Can you work these out from the drawing? Everything is in mm from the part's minimum corner. A direction names the side the tool comes from. Round coordinates to 2 decimals unless told otherwise and drop trailing zeros. Write each loop counter-clockwise with the first axis right and the second up, starting at its lowest first coordinate (ties: lowest second). Pieces come first, ordered by that corner, then holes. Notation, with made-up numbers: M 23.25,-13.5 L 36.25,-13.5 A24 cw 36.25,7.5 Z; hole C 16.5,-17.75 d9. An arc over 180 degrees is marked long. Use one line per item in the form item = value. Start each with the question number.
Q1. I want a section at A-A on y = 24. List the corners of the cut face in (x, z) for me.
Q2. I'm going to push flat-ended pins straight in: pin 1 Ø10 at (y, z) = (11, 7.5) entering from +X; pin 2 Ø2 at (y, z) = (27.5, 7) entering from +X; pin 3 Ø3 at (x, z) = (23.5, 8.5) entering from +Y (1 decimal). Where does each tip first touch, or does it pass through?
Q3. I want a section at C-C on z = 9.25. List the corners of the cut face in (x, y) for me, and give its area (3 significant figures).
Q4. I want a section at B-B on x = 23. List the corners of the cut face in (y, z) for me (1 decimal).
Q5. We'd pull the mould along X, two halves only. Please class the marked faces 3, 4 and 5: +X half, -X half, draft (parallel to the pull), parting line (faces both ways), or undercut.
Q6. For the marked faces 1 and 2, which set-ups out of +Z, -Z, +X, -X, +Y, -Y let a thin tool reach every point of the face, with its end or its side?
Q7. I need wall thicknesses on line 1 along X through (y, z) = (29.5, 8.5) (1 decimal); line 2 along X through (y, z) = (17, 10.25) (1 decimal); line 3 along Y through (x, z) = (19, 14.25). Which ranges of each line are inside material? Lowest first, please. Write a range as from..to.
Q8. I want a section at D-D on y = 13. List the corners of the cut face in (x, z) for me, and give its area (3 significant figures).
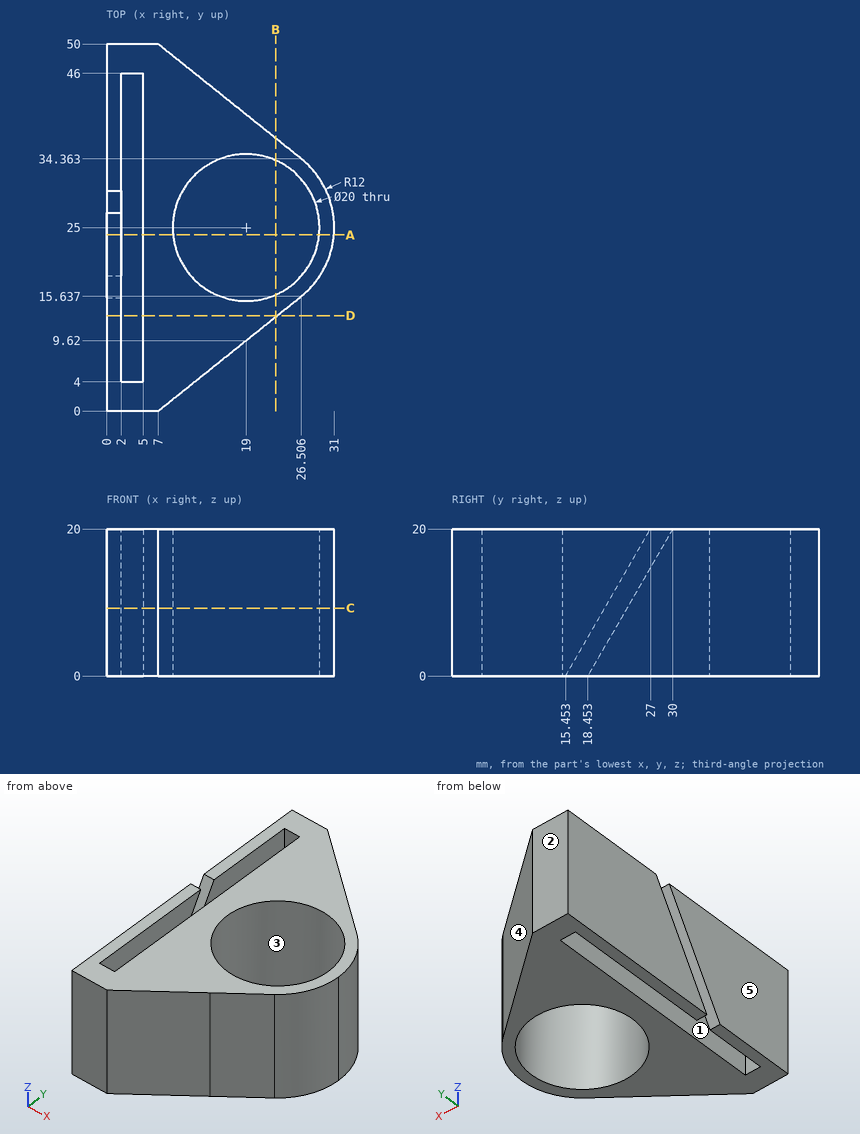
Reported:
q1.outline = M 0,0 L 2,0 L 2,9.61 L 0,9.61 Z; M 0,14.8 L 2,14.8 L 2,20 L 0,20 Z; M 5,0 L 9.05,0 L 9.05,20 L 5,20 Z; M 28.95,0 L 30.96,0 L 30.96,20 L 28.95,20 Z
q2.pin_1 = 26.94
q2.pin_2 = 30.91
q2.pin_3 = 38
q3.outline = M 0,0 L 7,0 L 26.51,15.64 A12 ccw 26.51,34.36 L 7,50 L 0,50 L 0,23.79 L 2,23.79 L 2,46 L 5,46 L 5,4 L 2,4 L 2,20.79 L 0,20.79 Z; hole C 19,25 d20
q3.area = 633 mm^2
q4.outline = M 12.8,0 L 15.8,0 L 15.8,20 L 12.8,20 Z; M 34.2,0 L 37.2,0 L 37.2,20 L 34.2,20 Z
q5.face_3 = undercut
q5.face_4 = +X half
q5.face_5 = -X half
q6.face_1 = +Z, -Z
q6.face_2 = +Z, -Z, +X, -X, +Y
q7.line_1 = 0..2, 5..10.1, 27.9..30.1
q7.line_2 = 0..2, 5..13, 25..27.9
q7.line_3 = 9.62..15, 35..40.38
q8.outline = M 0,0 L 2,0 L 2,20 L 0,20 Z; M 5,0 L 23.22,0 L 23.22,20 L 5,20 Z
q8.area = 404 mm^2
